Build history of the part. All positions in model axes, mm. Round coordinates to 2 decimals unless told otherwise and drop trailing zeros. Write each loop counter-clockwise with the first axis right and the second up, starting at its lowest first coordinate (ties: lowest second). Pieces come first, ordered by that corner, then holes. Notation, with made-up numbers: (23.5, -7) -> (41.5, -7) arc R8 cw to (41.5, -1) -> close; hole circle Ø8 at (-21.75, -15). An arc over 180 degrees is marked (long way). Return JSON: item names as keys, results as strings.
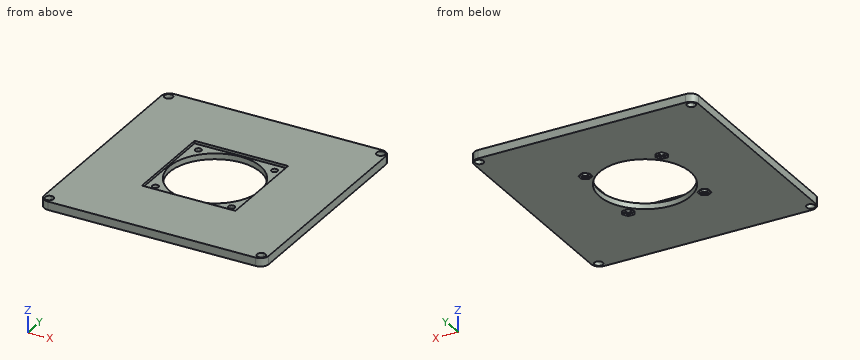
from build123d import *

# Parameters (mm, degrees)
F0_W             = 137.16
F0_H             = 137.16
F1_DEPTH         = 5.08
F2_R             = 5.08
F3_R             = 27.78125
F4_DEPTH         = 5.08
F5_W             = 57.15
F5_H             = 57.15
F6_DEPTH         = 1.5875
F8_DEPTH         = 3.4925
F8_COPIES_COUNT  = 4
F11_DEPTH        = 1.27
F11_COPIES_COUNT = 4
F13_DEPTH        = 5.08


# Not quite as in the source:
# - a pattern or mirror of a feature is missing from the dataset's text; its kind, count and spacing are read off the source's solid


with BuildPart() as f1:
    # F0 (on Top) → F1 (new body)
    with BuildSketch(Plane.XY):
        Rectangle(F0_W, F0_H)
    extrude(amount=F1_DEPTH)

    # F2
    f2_edges = [f1.edges().sort_by_distance(p)[0] for p in [
        (-68.58, -68.58, 2.54),
        (68.58, -68.58, 2.54),
        (68.58, 68.58, 2.54),
        (-68.58, 68.58, 2.54),
    ]]
    fillet(f2_edges, radius=F2_R)

    # F3 (on face) → F4 (cut, through all)
    with BuildSketch(Plane.XY.offset(5.08)):
        Circle(F3_R)
    extrude(amount=-F4_DEPTH, mode=Mode.SUBTRACT)

    # F5 (on face) → F6 (cut)
    with BuildSketch(Plane.XY.offset(5.08)):
        Rectangle(F5_W, F5_H)
    extrude(amount=-F6_DEPTH, mode=Mode.SUBTRACT)

    # F7 (on face) → F8 (cut, through all)
    with BuildSketch(Plane.XY.offset(3.4925)):
        with BuildLine():
            Line((21.9296104704, 21.9296104704), (24.6236873067, 24.6236873067))
            ThreePointArc((24.6236873067, 24.6236873067), (21.9296104704, 24.6236873067), (21.9296104704, 21.9296104704))
        make_face()
        with BuildLine():
            ThreePointArc((25.1816488886, 23.2766488886), (25.036639398, 24.0056608272), (24.6236873067, 24.6236873067))
            Line((24.6236873067, 24.6236873067), (21.9296104704, 21.9296104704))
            ThreePointArc((21.9296104704, 21.9296104704), (24.0056608272, 21.5166583791), (25.1816488886, 23.2766488886))
        make_face()
    f8 = extrude(amount=-F8_DEPTH, mode=Mode.SUBTRACT)

    # F8_copies: F8 ×4 about axis
    f8_copies_axis = Axis((0, 0, 0), (0, 0, 1))
    for i in range(1, F8_COPIES_COUNT):
        add(f8.rotate(f8_copies_axis, i * 360 / F8_COPIES_COUNT), mode=Mode.SUBTRACT)

    # F10 (on face) → F11 (cut)
    with BuildSketch(Plane(origin=(0, 0, 0), x_dir=(1, 0, 0), z_dir=(0, 0, -1))):
        Polygon((27.0866488886, 23.2766488886), (25.1816488886, 26.576205677), (21.3716488886, 26.576205677), (19.4666488886, 23.2766488886), (21.3716488886, 19.9770921002), (25.1816488886, 19.9770921002), align=None)
    f11 = extrude(amount=-F11_DEPTH, mode=Mode.SUBTRACT)

    # F11_copies: F11 ×4 about axis
    f11_copies_axis = Axis((0, 0, 0), (0, 0, 1))
    for i in range(1, F11_COPIES_COUNT):
        add(f11.rotate(f11_copies_axis, i * 360 / F11_COPIES_COUNT), mode=Mode.SUBTRACT)

    # F12 (on face) → F13 (cut, through all)
    with BuildSketch(Plane.XY.offset(5.08)):
        with BuildLine():
            Line((-64.77, 64.77), (-62.23, 64.77))
            ThreePointArc((-62.23, 64.77), (-66.5660512242, 66.5660512242), (-64.77, 62.23))
            Line((-64.77, 62.23), (-64.77, 64.77))
        make_face()
        with BuildLine():
            ThreePointArc((-64.77, 62.23), (-62.9739487758, 62.9739487758), (-62.23, 64.77))
            Line((-62.23, 64.77), (-64.77, 64.77))
            Line((-64.77, 64.77), (-64.77, 62.23))
        make_face()
        with BuildLine():
            Line((-64.77, -64.77), (-64.77, -62.23))
            ThreePointArc((-64.77, -62.23), (-66.5660512242, -66.5660512242), (-62.23, -64.77))
            Line((-62.23, -64.77), (-64.77, -64.77))
        make_face()
        with BuildLine():
            ThreePointArc((-62.23, -64.77), (-62.9739487758, -62.9739487758), (-64.77, -62.23))
            Line((-64.77, -62.23), (-64.77, -64.77))
            Line((-64.77, -64.77), (-62.23, -64.77))
        make_face()
        with BuildLine():
            ThreePointArc((67.31, -64.77), (66.5660512242, -62.9739487758), (64.77, -62.23))
            Line((64.77, -62.23), (64.77, -64.77))
            Line((64.77, -64.77), (62.23, -64.77))
            ThreePointArc((62.23, -64.77), (64.77, -67.31), (67.31, -64.77))
        make_face()
        with BuildLine():
            Line((64.77, -64.77), (64.77, -62.23))
            ThreePointArc((64.77, -62.23), (62.9739487758, -62.9739487758), (62.23, -64.77))
            Line((62.23, -64.77), (64.77, -64.77))
        make_face()
        with BuildLine():
            Line((64.77, 64.77), (62.23, 64.77))
            ThreePointArc((62.23, 64.77), (62.9739487758, 62.9739487758), (64.77, 62.23))
            Line((64.77, 62.23), (64.77, 64.77))
        make_face()
        with BuildLine():
            ThreePointArc((67.31, 64.77), (64.77, 67.31), (62.23, 64.77))
            Line((62.23, 64.77), (64.77, 64.77))
            Line((64.77, 64.77), (64.77, 62.23))
            ThreePointArc((64.77, 62.23), (66.5660512242, 62.9739487758), (67.31, 64.77))
        make_face()
    extrude(amount=-F13_DEPTH, mode=Mode.SUBTRACT)


solid = f1.part
Q1. Saw through at A-A on x = 0. List the corners of the cut face in (y, z) (1 decimal), then the cut area to 3 significant figures.
Verdict:
{"outline": "(-68.6, 0) -> (-27.8, 0) -> (-27.8, 3.5) -> (-28.6, 3.5) -> (-28.6, 5.1) -> (-68.6, 5.1) -> close; (27.8, 0) -> (68.6, 0) -> (68.6, 5.1) -> (28.6, 5.1) -> (28.6, 3.5) -> (27.8, 3.5) -> close", "area": "412 mm²"}
Q2. Pin check, flat tip, straight feed: pin 1 Ø3.5 at (x, y) = (25, -21.5) entering from -Z. Stop position of the tip, or through.
Verdict:
{"pin 1": "stops at z = 0"}
Q3. Saw through at B-B on y = -6. List the corners of the cut face in (x, z) (1 decimal).
Verdict:
{"outline": "(-68.6, 0) -> (-27.1, 0) -> (-27.1, 3.5) -> (-28.6, 3.5) -> (-28.6, 5.1) -> (-68.6, 5.1) -> close; (27.1, 0) -> (68.6, 0) -> (68.6, 5.1) -> (28.6, 5.1) -> (28.6, 3.5) -> (27.1, 3.5) -> close"}
Q4. Wall check: L1, parallel to X at y = 64.77, z = 1.15; L2, parallel to Y at x = -10.5, z = 4.8 (3 decimals); L3, parallel to X at y = -20.5, z = 0.7. Give the ranges that are in metal, low to high.
Verdict:
{"L1": "x = -68.42 to -67.31, -62.23 to 62.23, 67.31 to 68.42", "L2": "y = -68.58 to -28.575, 28.575 to 68.58", "L3": "x = -68.58 to -25.07, -21.49 to -18.75, 18.75 to 21.07, 25.48 to 68.58"}
